Input: dimensioned drawing with shaded views. Units: mm. Origin: part minimum x, y, z. Coordinates: 2 decimals unless noted, no trailing zeros. Write each loop counter-clockwise with the first axis right and the second up, starting at its lowest first coordinate (ties: lowest second). Pieces come first, ordered by that corner, then holes. Notation, with made-up numbers: (72.25, 85.5) -> (119.25, 85.5) arc R23 ccw to (119.25, 122.5) -> close; hole circle Ø5 at (-26.5, -31). An arc over 180 degrees is marked (long way). One line per item, written item: value. Start each with the question number.
1. Section query A-A, the plane x = 40. Output: boundary loops of the cut face in (y, z).
2. Section query B-B, the plane y = 51. Output: boundary loops of the cut face in (x, z), and give its area (3 significant figures).
3. Section query D-D, the plane x = 7. Output: boundary loops of the cut face in (y, z).
4. First-contact query: P1, Ø5, axis at x = 11.5, y = 38.5, coming from the -Z side. Flat tip, straight axial feed; report the tip coordinate or a pass-through.
5. Section query C-C, the plane z = 0.6. Output: boundary loops of the cut face in (x, y), and give its area (3 significant figures).
6. Line query: line 1 (Y direction, x = 73, z = 0.35); line 2 (Y direction, x = 40, z = 0.5); line 3 (Y direction, x = 71, z = 0.85). Output: solid intervals per line, ascending.
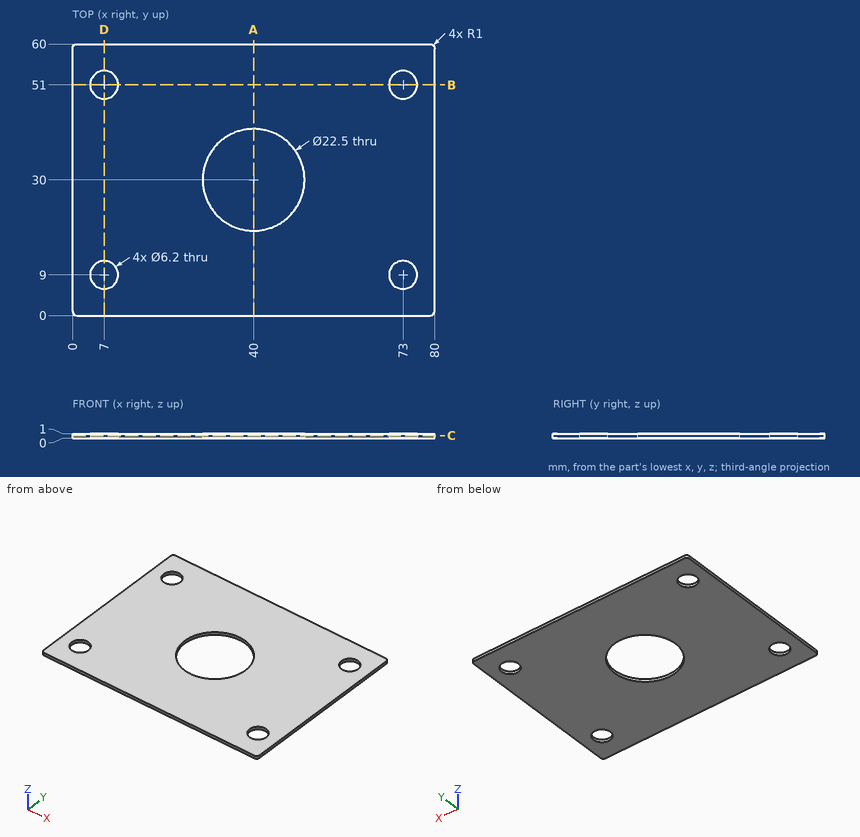
Computed values:
1. outline: (0, 0) -> (18.75, 0) -> (18.75, 1) -> (0, 1) -> close; (41.25, 0) -> (60, 0) -> (60, 1) -> (41.25, 1) -> close
2. outline: (0, 0) -> (3.9, 0) -> (3.9, 1) -> (0, 1) -> close; (10.1, 0) -> (69.9, 0) -> (69.9, 1) -> (10.1, 1) -> close; (76.1, 0) -> (80, 0) -> (80, 1) -> (76.1, 1) -> close
2. area: 67.6 mm²
3. outline: (0, 0) -> (5.9, 0) -> (5.9, 1) -> (0, 1) -> close; (12.1, 0) -> (47.9, 0) -> (47.9, 1) -> (12.1, 1) -> close; (54.1, 0) -> (60, 0) -> (60, 1) -> (54.1, 1) -> close
4. P1: stops at z = 0
5. outline: (0, 1) arc R1 ccw to (1, 0) -> (79, 0) arc R1 ccw to (80, 1) -> (80, 59) arc R1 ccw to (79, 60) -> (1, 60) arc R1 ccw to (0, 59) -> close; hole circle Ø6.2 at (7, 9); hole circle Ø6.2 at (7, 51); hole circle Ø22.5 at (40, 30); hole circle Ø6.2 at (73, 9); hole circle Ø6.2 at (73, 51)
5. area: 4,280 mm²
6. line 1: y = 0 to 5.9, 12.1 to 47.9, 54.1 to 60
6. line 2: y = 0 to 18.75, 41.25 to 60
6. line 3: y = 0 to 6.63, 11.37 to 48.63, 53.37 to 60
